Work out the finished part from the listing and answer in its coordinate system (mm). A direction names the side the tool comes from. Coordinates: 2 decimals unless noted, no trailing zeros. Order: outer loops, then holes, each group sorted by start corner. A loop starts at its lowest first (then second) coordinate and runs counter-clockwise, first axis right, second up. Notation, with made-up numbers: (0, -29) -> (34, -29) arc R32 ccw to (34, 8) -> close; hole circle Ø4 at (20, 62.5). An arc over 180 degrees is marked (long way). Answer as CSV lines item,"result". Start each with the question number.
Item 1: Section B-B (x = -10) is taken. Write down the section's boundary in (y, z) (3 decimals).
Item 2: Which of the six approach directions +Z, -Z, +X, -X, +Y, -Y give full straight-line access (tool end or side, diameter ignored) to faces 1 (the face through (-14, 0, 23.749)), 2 (the face through (0, 2.491, 11)), 3 (the face through (-0.116, -14.534, 22.976))?
Item 3: Section C-C (y = -4) is taken. Write down the section's boundary in (x, z) (3 decimals), then the cut area to 3 significant figures.
Item 4: Section A-A (z = 13.5) is taken. Write down the section's boundary in (x, y) (3 decimals).
Item 5: For a pull along X with two mould halves and no side action, classify faces 4 (the face through (0, 3, 0)), 5 (the face through (-7.702, -6, 11)), 6 (the face through (0.54, 12.933, 22.976)), 7 (the face through (12.786, 0.086, 22.976)) as pulls with the +X half, pulls with the -X half, needs draft (parallel to the pull), parting line crosses it, or undercut.
Item 6: Section D-D (x = 0) is taken. Write down the section's boundary in (y, z) (3 decimals).
Item 7: Each of these flat-tipped pins is pushed along its axis until it touches: pin 1 Ø5 at (y, z) = (6, 8) entering from -X; pin 2 Ø3 at (x, z) = (9, 5.5) entering from +Y; pin 3 Ø1.4 at (y, z) = (1, 7) entering from -X; pin 4 Ø1 at (x, y) = (-3.5, 0.5) entering from +Z. Where does it stop, or does it pass through?
Item 8: Straight lines are drawn through the part: L1, parallel to Y at x = -0.5, z = 16.5; L2, parallel to Y at x = 4, z = 18; L3, parallel to Z at x = -10.5, y = -3 (3 decimals). For each, find the intervals that lie inside material, in ascending order.
```python
from build123d import *

# Parameters (mm, degrees)
F0_R     = 15.875
F1_DEPTH = 22.225
F3_R     = 0.889
F5_DEPTH = 23.749
F7_W     = 21.828934
F7_H     = 4.78795
F7_W_2   = 15.322826
F7_H_2   = 4.7625
F6_DEPTH = 22.225


with BuildPart() as f1:
    # F0 (on Top) → F1 (new body)
    with BuildSketch(Plane.XY):
        Circle(F0_R)
    extrude(amount=F1_DEPTH)

    # F3 (on face) → F5 (join)
    with BuildSketch(Plane(origin=(0, 0, 0), x_dir=(1, 0, 0), z_dir=(0, 0, -1))):
        with Locations((0, 13.652203)):
            Circle(F3_R)
        with Locations((-13.659894, -0.015021)):
            Circle(F3_R)
        with Locations((0.062219, -13.682245)):
            Circle(F3_R)
        with Locations((13.674476, -0.124876)):
            Circle(F3_R)
    extrude(amount=-F5_DEPTH)

    # F7 (on face) → F6 (cut)
    with BuildSketch(Plane.XY.offset(22.225)):
        with Locations((0.014928, 0.097281)):
            Rectangle(F7_W, F7_H)
        with Locations((-0.040691, 5.869923)):
            Rectangle(F7_W_2, F7_H_2)
        with Locations((-0.040691, -5.869923)):
            Rectangle(F7_W_2, F7_H_2)
    extrude(amount=-F6_DEPTH, mode=Mode.SUBTRACT)


solid = f1.part
```
Checked values:
1,outline,"(-12.329, 0) -> (-2.297, 0) -> (-2.297, 22.225) -> (-12.329, 22.225) -> close; (2.491, 0) -> (12.329, 0) -> (12.329, 22.225) -> (2.491, 22.225) -> close"
2,face 1,"+Z, +X, -X, +Y, -Y"
2,face 2,"+Z, -Z"
2,face 3,"+Z"
3,outline,"(-15.363, 0) -> (-7.702, 0) -> (-7.702, 22.225) -> (-15.363, 22.225) -> close; (7.621, 0) -> (15.363, 0) -> (15.363, 22.225) -> (7.621, 22.225) -> close"
3,area,"342 mm^2"
4,outline,"circle Ø31.75 at (0, 0); hole (-10.9, -2.297) -> (10.929, -2.297) -> (10.929, 2.491) -> (-10.9, 2.491) -> close; hole (-7.702, -8.251) -> (7.621, -8.251) -> (7.621, -3.489) -> (-7.702, -3.489) -> close; hole (-7.702, 3.489) -> (7.621, 3.489) -> (7.621, 8.251) -> (-7.702, 8.251) -> close"
5,face 4,"needs draft"
5,face 5,"undercut"
5,face 6,"parting line crosses it"
5,face 7,"undercut"
6,outline,"(-15.875, 0) -> (-8.251, 0) -> (-8.251, 22.225) -> (-12.763, 22.225) -> (-12.763, 23.749) -> (-14.541, 23.749) -> (-14.541, 22.225) -> (-15.875, 22.225) -> close; (-3.489, 0) -> (-2.297, 0) -> (-2.297, 22.225) -> (-3.489, 22.225) -> close; (2.491, 0) -> (3.489, 0) -> (3.489, 22.225) -> (2.491, 22.225) -> close; (8.251, 0) -> (15.875, 0) -> (15.875, 22.225) -> (14.569, 22.225) -> (14.569, 23.749) -> (12.795, 23.749) -> (12.795, 22.225) -> (8.251, 22.225) -> close"
7,pin 1,"stops at x = -15.48"
7,pin 2,"stops at y = 13.99"
7,pin 3,"stops at x = -15.87"
7,pin 4,"passes through"
8,L1,"y = -15.87 to -8.25, -3.49 to -2.3, 2.49 to 3.49, 8.25 to 15.87"
8,L2,"y = -15.36 to -8.25, -3.49 to -2.3, 2.49 to 3.49, 8.25 to 15.36"
8,L3,"z = 0 to 22.225"
